Read the model definition and answer for the solid it produces. Units are mm, in the model's axes. A direction names the side the tool comes from. Give positions to 0.01 mm unless a question says otherwise; leave off trailing zeros. Order: outer loops, then holes, each group sorted by start corner. A loop starts at its lowest first (then second) coordinate and runs counter-clockwise, first axis right, second up.
```python
from build123d import *

# Parameters (mm, degrees)
SKETCH_1_W      = 40
SKETCH_1_H      = 20
SKETCH_1_R      = 1.5
EXTRUDE_1_DEPTH = 4
SKETCH_2_W      = 40
SKETCH_2_H      = 25
SKETCH_2_R      = 1.5
EXTRUDE_2_DEPTH = 4


with BuildPart() as part:
    # Эскиз1 → Бобышка-Вытянуть1 (new body)
    with BuildSketch(Plane.XY):
        Rectangle(SKETCH_1_W, SKETCH_1_H)
        with Locations((-16, 0)):
            Circle(SKETCH_1_R, mode=Mode.SUBTRACT)
        with Locations(Location((16, 0, 0), (0, 0, 180))):
            Circle(SKETCH_1_R, mode=Mode.SUBTRACT)
    extrude(amount=EXTRUDE_1_DEPTH)

    # Эскиз2 → Бобышка-Вытянуть2 (add)
    with BuildSketch(Plane.XZ.offset(10)):
        with Locations((0, 16.5)):
            Rectangle(SKETCH_2_W, SKETCH_2_H)
        with Locations(Location((-7.27406928, 21.5, 0), (0, 0, 270))):
            Circle(SKETCH_2_R, mode=Mode.SUBTRACT)
        with Locations(Location((-7.27406928, 11.5, 0), (0, 0, 270))):
            Circle(SKETCH_2_R, mode=Mode.SUBTRACT)
    extrude(amount=-EXTRUDE_2_DEPTH)


solid = part.part
```
1) The part is cut by section D-D on x = -1.5. Determine the outline of the cut face in (y, z).
Final values:
outline: (-10, 0) - (10, 0) - (10, 4) - (-6, 4) - (-6, 29) - (-10, 29) - close
2) The part is cut by section C-C on z = 11.5. Determine the outline of the cut face in (x, y), and give its area (3 significant figures).
Final values:
outline: (-20, -10) - (-8.77, -10) - (-8.77, -6) - (-20, -6) - close; (-5.77, -10) - (20, -10) - (20, -6) - (-5.77, -6) - close
area: 148 mm2
3) Consider L1, parallel to X at y = -8.4, z = 11.5; L2, parallel to Y at x = 16, z = 2.8; L3, parallel to Z at x = -16, y = 7.5. Determine where each line is inside the solid, lowest interval first.
Final values:
L1: x = -20 to -8.77, -5.77 to 20
L2: y = -10 to -1.5, 1.5 to 10
L3: z = 0 to 4
4) The part is cut by section A-A on x = -16. Determine the outline of the cut face in (y, z).
Final values:
outline: (-10, 0) - (-1.5, 0) - (-1.5, 4) - (-6, 4) - (-6, 29) - (-10, 29) - close; (1.5, 0) - (10, 0) - (10, 4) - (1.5, 4) - close
5) The part is cut by section B-B on y = 0. Determine the outline of the cut face in (x, z), and give its area (3 significant figures).
Final values:
outline: (-20, 0) - (-17.5, 0) - (-17.5, 4) - (-20, 4) - close; (-14.5, 0) - (14.5, 0) - (14.5, 4) - (-14.5, 4) - close; (17.5, 0) - (20, 0) - (20, 4) - (17.5, 4) - close
area: 136 mm2
6) For a pull along Z with two mould halves and no side action, classify faces 3 (the face through (17.5, -0.07, 1.97)), 4 (the face through (-5.787, -8.028, 11.695)), 5 (the face through (0, -8, 29)) as released by +Z, released by -Z, zero draft, split by the parting line, or undercut.
Final values:
face 3: zero draft
face 4: undercut
face 5: released by +Z
7) Given pin 1 (5 mm diameter, centred on x = -0.5, y = 3, fed in from +Z); pin 2 (12.5 mm diameter, centred on x = -9.5, z = 22, fed in from +Y), each flat-ended and moving along its own axis, determine where each tip first touches the part or whether it passes through.
Final values:
pin 1: stops at z = 4
pin 2: stops at y = -6
8) A tool of negligible diameter and unlimited length cuts with its end or side. For faces 1 (the face through (0, -6, 17)), 2 (the face through (-6.26, -8.028, 22.606)), from which of +Z, -Z, +X, -X, +Y, -Y can it reach the whole face along a straight path? Write none if from no direction.
Final values:
face 1: +Z, +X, -X, +Y
face 2: +Y, -Y
